Can you work these out from the model? Positions are in its coordinate system, mm. Face numbers are marked on the shaded views. Give positions to 0.01 mm unless a question says otherwise; leave off trailing zeros. Order: outer loops, then holes, each group sorted by start corner. A loop starts at its lowest first (then second) coordinate and runs counter-clockwise, first axis right, second up.
Item 1: I want a section at A-A, the plane x = 16. Write out the boundary of the cut face in (y, z).
Item 2: I want a section at B-B, the plane z = 1.75. Write out the boundary of the cut face in (x, y), then the cut area to 3 significant figures.
Item 3: I'm going to push flat-ended pins straight in: pin 1 Ø4 at (x, y) = (0, 6.731) entering from +Z; pin 2 Ø5 at (x, y) = (-16, 34.11) entering from -Z; pin 3 Ø2 at (x, y) = (0, 29.98) entering from -Z; pin 4 Ø1 at (y, z) = (15.5, 0.5) entering from +X. Where does each tip first touch, or does it pass through?
Item 4: If we mould it in two halves opening along Y, with no side actions, what happens to the marked faces 1, 2, 3 and 4? For each: +Y half, -Y half, draft (parallel to the pull), parting line (faces both ways), or undercut.
Item 5: I want a section at C-C, the plane y = 18.5. Write out the boundary of the cut face in (x, z).
Item 6: If I drill on line 1 along Y through (x, z) = (0, 5.6); line 2 along Y through (x, z) = (0, 1.5); line 3 along X through (y, z) = (9, 2.75), over which ranges is the centre line in solid material (lowest first)?
Item 7: I want a section at D-D, the plane y = 7.5. Write out the boundary of the cut face in (x, z).
Autodesk Inventor part; units mm, degrees
ref_plane "YZ Plane" through (0, 0, 0) normal (1, 0, 0) x (0, 1, 0)
ref_plane "XZ Plane" through (0, 0, 0) normal (0, 1, 0) x (-1, 0, 0)
ref_plane "XY Plane" through (0, 0, 0) normal (0, 0, 1) x (1, 0, 0)
ref_plane "Work Plane7" through (21.5, 42.1122, 7.5565) normal (0, 0, -1) x (0, 1, 0)
sketch "Sketch4" plane through (21.5, 42.1122, 7.5565) normal (0, 0, -1) x (0, 1, 0)
  line L0 (-42.1122, -17.69) -> (-42.1122, -25.31) construction
  line L1 (0, 0) -> (0, -43) construction
  line L2 (-528, -43) -> (0, -43) construction
  line L3 (-528, 0) -> (0, 0) construction
  line L4 (-42.1122, -43) -> (0, -43)
  line L5 (0, -43) -> (0, 0)
  line L6 (0, 0) -> (-42.1122, 0)
  line L7 (-42.1122, 0) -> (-42.1122, -43)
  circle A0 centre (-8, -5.5) radius 2
  circle A1 centre (-32, -5.5) radius 2
  circle A2 centre (-8, -37.5) radius 2
  circle A3 centre (-32, -37.5) radius 2
  point P0 (-42.1122, -21.5)
extrude "Extrusion4" add sketch "Sketch4" along normal blind 6.35
ref_plane "Work Plane6" through (0, 0, 0) normal (0, 0, 1) x (1, 0, 0)
sketch "Sketch5" plane through (0, 0, 0) normal (0, 0, 1) x (1, 0, 0)
  line L0 (3.1132, 0) -> (3.1132, 33.02) construction
  line L1 (-3.1132, 0) -> (-3.1132, 33.02) construction
  line L2 (3.14, 32.92) -> (-3.14, 32.92) construction
  line L3 (-21.5, 0) -> (21.5, 0) construction
  line L4 (3.1132, 0) -> (-3.14, 0)
  line L5 (-3.14, 0) -> (-3.14, 32.92)
  line L6 (-3.14, 32.92) -> (3.1132, 32.92)
  line L7 (3.1132, 32.92) -> (3.1132, 0)
  arc A0 (-0.0115, 8.4836) -> (1.2335, 7.976) centre (0, 6.731) ccw construction
  spline S0 degree 3 poles (-3.9963, 27.1983) (-3.9282, 27.0439) (-3.8705, 26.8672) (-3.7787, 26.4733) (-3.747, 26.2579) (-3.7229, 25.8912) (-3.7161, 25.6578) (-3.7657, 25.2017) (-3.8042, 25.0235) (-3.9064, 24.7384) (-3.9674, 24.6297) (-4.0735, 24.5156) (-4.1125, 24.4855) (-4.225, 24.4328) (-4.3003, 24.4339) (-4.4555, 24.5079) (-4.5339, 24.5853) (-4.6625, 24.7855) (-4.7303, 24.9172) (-4.8354, 25.2648) (-4.8698, 25.4348) (-4.9129, 25.8035) (-4.9196, 25.9997) (-4.906, 26.2838) (-4.8978, 26.3737) (-4.8628, 26.6198) (-4.8272, 26.7652) (-4.7302, 27.0244) (-4.6681, 27.1326) (-4.5976, 27.2088) knots 0.000001 0.000001 0.000001 0.000001 0.061283 0.061283 0.126502 0.126502 0.171802 0.171802 0.206523 0.206523 0.238722 0.238722 0.255636 0.255636 0.285543 0.285543 0.317605 0.317605 0.342807 0.342807 0.362438 0.362438 0.383231 0.383231 0.393319 0.393319 0.411548 0.411548 0.431083 0.431083 0.431083 0.431083 construction
  circle A1 centre (0, 6.731) radius 1.778 construction
  circle A2 centre (-0.0134, 32.92) radius 1.778 construction
  point P0 (0, 0)
  dimension "d10" = 3.556
  dimension "d11" = 3.556
extrude "Extrusion5" add sketch "Sketch5" along normal up to surface (1.2065 mm away)
sketch "Sketch6" plane through (21.5, 42.1122, 7.5565) normal (0, 0, 1) x (1, 0, 0)
  arc A0 (-21.5115, -33.6287) -> (-20.2665, -34.1362) centre (-21.5, -35.3812) ccw construction
  arc A1 (-21.5115, -10.3793) -> (-20.2665, -10.8868) centre (-21.5, -12.1318) ccw construction
  point P0 (-21.5, -42.1122)
hole "Hole2" at (0, 6.731, 7.5565) at (0, 29.9804, 7.5565) direction (0, 0, -1) diameter 3.556 end through all
ref_plane "Work Plane8" through (21.5, 42.1122, 7.5565) normal (0, 0, 1) x (1, 0, 0)
sketch "Sketch7" plane through (21.5, 42.1122, 7.5565) normal (0, 0, 1) x (1, 0, 0)
  circle A0 centre (-21.5, -12.1318) radius 1.778
  circle A1 centre (-21.5, -12.1318) radius 5.08
  circle A2 centre (-21.5, -35.3812) radius 1.778
  circle A3 centre (-21.5, -35.3812) radius 5.08
  point P0 (-21.5, -42.1122)
  dimension "d28" = 10.16
  dimension "d29" = 10.16
extrude "Extrusion6" cut sketch "Sketch7" against normal blind 5.08
properties part number "LeadScrewNutCoupler"
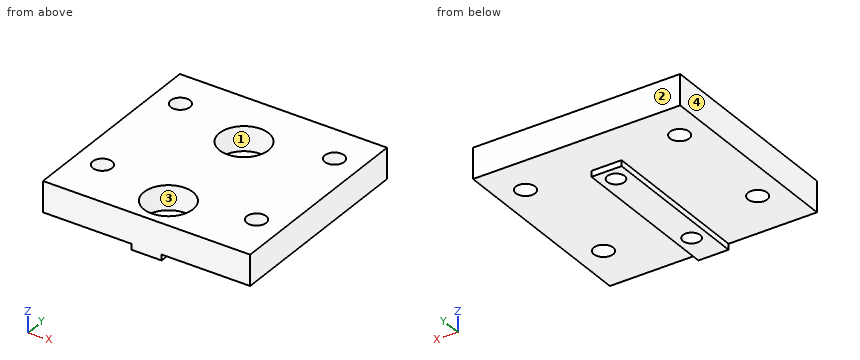
Results list:
1. outline: (0, 1.21) - (8.11, 1.21) - (8.11, 7.56) - (0, 7.56) - close; (12.11, 1.21) - (32.11, 1.21) - (32.11, 7.56) - (12.11, 7.56) - close; (36.11, 1.21) - (42.11, 1.21) - (42.11, 7.56) - (36.11, 7.56) - close
2. outline: (-21.5, 0) - (21.5, 0) - (21.5, 42.11) - (-21.5, 42.11) - close; hole circle Ø4 at (-16, 10.11); hole circle Ø4 at (-16, 34.11); hole circle Ø3.56 at (0, 6.73); hole circle Ø3.56 at (0, 29.98); hole circle Ø4 at (16, 10.11); hole circle Ø4 at (16, 34.11)
2. area: 1,740 mm2
3. pin 1: stops at z = 2.48
3. pin 2: stops at z = 1.21
3. pin 3: passes through
3. pin 4: stops at x = 3.11
4. face 1: undercut
4. face 2: +Y half
4. face 3: undercut
4. face 4: draft
5. outline: (-21.5, 1.21) - (-3.14, 1.21) - (-3.14, 0) - (3.11, 0) - (3.11, 1.21) - (21.5, 1.21) - (21.5, 7.56) - (-21.5, 7.56) - close
6. line 1: y = 0 to 1.65, 11.81 to 24.9, 35.06 to 42.11
6. line 2: y = 0 to 4.95, 8.51 to 28.2, 31.76 to 42.11
6. line 3: x = -21.5 to -17.66, -14.34 to -4.55, 4.55 to 14.34, 17.66 to 21.5
7. outline: (-21.5, 1.21) - (-3.14, 1.21) - (-3.14, 0) - (-1.6, 0) - (-1.6, 2.48) - (-5.02, 2.48) - (-5.02, 7.56) - (-21.5, 7.56) - close; (1.6, 0) - (3.11, 0) - (3.11, 1.21) - (21.5, 1.21) - (21.5, 7.56) - (5.02, 7.56) - (5.02, 2.48) - (1.6, 2.48) - close
